```python
from build123d import *

# Parameters (mm, degrees)
F1_DEPTH  = 100
F2_R      = 3
F3_DEPTH  = 105.001
F4_W      = 66
F4_H      = 70
F5_DEPTH  = 25
F6_W      = 2
F6_H      = 15
F7_DEPTH  = 29
F8_W      = 15
F8_H      = 2
F9_DEPTH  = 3
F10_W     = 15
F10_H     = 2
F11_DEPTH = 3
F12_R     = 1
F13_R     = 2
F14_R     = 5


with BuildPart() as f1:
    # F0 (on Front) → F1 (new body)
    with BuildSketch(Plane.XZ):
        Polygon((105, 26), (0, 26), (0, 0), (2, 0), (2, 24), (103, 24), (103, 0), (105, 0), align=None)
    extrude(amount=F1_DEPTH)

    # F2 (on face) → F3 (cut, through all)
    with BuildSketch(Plane.YZ.offset(105)):
        with Locations((-7, 5)):
            Circle(F2_R)
        with Locations((-49, 5)):
            Circle(F2_R)
    extrude(amount=-F3_DEPTH, mode=Mode.SUBTRACT)

    # F4 (on face) → F5 (cut)
    with BuildSketch(Plane.XY.offset(26)):
        with Locations((52.5, -35)):
            Rectangle(F4_W, F4_H)
    extrude(amount=-F5_DEPTH, mode=Mode.SUBTRACT)

    # F6 (on face) → F7 (join)
    with BuildSketch(Plane.XY.offset(26)):
        with Locations((18.5, -7.5)):
            Rectangle(F6_W, F6_H)
        with Locations((18.5, -52.5)):
            Rectangle(F6_W, F6_H)
        with Locations((86.5, -7.5)):
            Rectangle(F6_W, F6_H)
        with Locations((86.5, -52.5)):
            Rectangle(F6_W, F6_H)
    extrude(amount=F7_DEPTH)

    # F8 (on face) → F9 (join)
    with BuildSketch(Plane.YZ.offset(19.5)):
        with Locations((-52.5, 54)):
            Rectangle(F8_W, F8_H)
        with Locations((-7.5, 54)):
            Rectangle(F8_W, F8_H)
    extrude(amount=F9_DEPTH)

    # F10 (on face) → F11 (join)
    with BuildSketch(Plane(origin=(85.5, 0, 0), x_dir=(0, -1, 0), z_dir=(-1, 0, 0))):
        with Locations((7.5, 54)):
            Rectangle(F10_W, F10_H)
        with Locations((52.5, 54)):
            Rectangle(F10_W, F10_H)
    extrude(amount=F11_DEPTH)

    # F12
    f12_edges = [f1.edges().sort_by_distance(p)[0] for p in [
        (2, -50, 24),
        (103, -50, 24),
        (17.5, -7.5, 26),
        (18.5, -15, 26),
        (17.5, -52.5, 26),
        (18.5, -60, 26),
        (18.5, -45, 26),
        (86.5, -60, 26),
        (87.5, -52.5, 26),
        (86.5, -15, 26),
        (87.5, -7.5, 26),
        (86.5, -45, 26),
    ]]
    fillet(f12_edges, radius=F12_R)

    # F13
    f13_edges = [f1.edges().sort_by_distance(p)[0] for p in [
        (0, -50, 26),
        (105, -50, 26),
    ]]
    fillet(f13_edges, radius=F13_R)

    # F14
    f14_edges = [f1.edges().sort_by_distance(p)[0] for p in [
        (85.5, -70, 25),
        (19.5, -70, 25),
    ]]
    fillet(f14_edges, radius=F14_R)


solid = f1.part
```
Can you work these out from the model? Positions are in its coordinate system, mm. A direction names the side the tool comes from. Round coordinates to 2 decimals unless told otherwise and drop trailing zeros. Loops run counter-clockwise (first coordinate to the right, second up) from the corner with the lowest first, then second, coordinate; pieces in that order, holes last.
Item 1: Which directions (+Z, -Z, +X, -X, +Y, -Y) give clear straight access to the entire face, cutting with the end or side of a thin tool? Please do faces 1 (the flat face through (19, -15, 41)), 2 (the flat face through (87.5, -53, 41)), 3 (the flat face through (86, -60, 41)).
Item 2: Please list where these lines run through material, in increasing order: L1, parallel to X at y = -86.5, z = 17; L2, parallel to X at y = -54.5, z = 35; L3, parallel to Z at x = 104.35, y = -49.
Item 3: Suppose I cut it at A-A, the plane z = 29.5. Write out the boundary of the cut face in (x, y).
Item 4: If we mould it in two halves opening along X, with no side actions, what happens to faces 4 (the flat face through (86, -15, 41)), 5 (the flat face through (0, -49, 12)), 6 (the flat face through (87.5, -8, 41)), 7 (the flat face through (2, -49, 11))? For each: +X half, -X half, draft (parallel to the pull), parting line (faces both ways), or undercut.
Item 5: Will these pins go through, and if not, where does the flat tip stop? pin 1 Ø1.5 at (x, y) = (84, -4) entering from -Z; pin 2 Ø1 at (y, z) = (-14, 29) entering from +X; pin 3 Ø10 at (x, y) = (19.5, -33.5) entering from -Z.
Item 6: Suppose I cut it at C-C, the plane z = 5. Write out the boundary of the cut face in (x, y), then the cut area to 3 significant figures.
Item 7: Suppose I cut it at D-D, the plane y = -7. State how many separate pieces and enclosed holes the cut face has, then the cut area to 3 significant figures.
Item 8: Suppose I cut it at B-B, the plane y = -19.5. Write out the boundary of the cut face in (x, z).
Reported:
1. face 1: +Z, +X, -X
1. face 2: +Z, +X, +Y, -Y
1. face 3: +Z, +X, -X, -Y
2. L1: x = 0 to 2, 103 to 105
2. L2: x = 17.5 to 19.5, 85.5 to 87.5
2. L3: z = 0 to 2, 8 to 25.48
3. outline: (17.5, -60) - (19.5, -60) - (19.5, -45) - (17.5, -45) - close; (17.5, -15) - (19.5, -15) - (19.5, 0) - (17.5, 0) - close; (85.5, -60) - (87.5, -60) - (87.5, -45) - (85.5, -45) - close; (85.5, -15) - (87.5, -15) - (87.5, 0) - (85.5, 0) - close
4. face 4: draft
4. face 5: -X half
4. face 6: +X half
4. face 7: undercut
5. pin 1: stops at z = 53
5. pin 2: stops at x = 87.5
5. pin 3: stops at z = 24
6. outline: (0, -100) - (2, -100) - (2, -52) - (0, -52) - close; (0, -46) - (2, -46) - (2, -10) - (0, -10) - close; (0, -4) - (2, -4) - (2, 0) - (0, 0) - close; (103, -100) - (105, -100) - (105, -52) - (103, -52) - close; (103, -46) - (105, -46) - (105, -10) - (103, -10) - close; (103, -4) - (105, -4) - (105, 0) - (103, 0) - close
6. area: 352 mm2
7. separate pieces: 4
7. enclosed holes: 0
7. area: 277 mm2
8. outline: (0, 0) - (2, 0) - (2, 23) arc R1 cw to (3, 24) - (19.5, 24) - (19.5, 26) - (2, 26) arc R2 ccw to (0, 24) - close; (85.5, 24) - (102, 24) arc R1 cw to (103, 23) - (103, 0) - (105, 0) - (105, 24) arc R2 ccw to (103, 26) - (85.5, 26) - close
